Part model, mm, in its own coordinate system. Coordinates: 2 decimals unless noted, no trailing zeros. Order: outer loops, then holes, each group sorted by start corner. A loop starts at its lowest first (then second) coordinate and runs counter-clockwise, first axis right, second up.
1) Wall check: L1, parallel to Z at x = -0.5, y = 1; L2, parallel to Z at x = -1.25, y = -0.5; L3, parallel to X at y = -0.5, z = 26. Give the ranges that are in metal, low to high.
2) Cut at C-C (x = -0.5). List the corners of the cut face in (y, z), and give its area (3 significant figures).
3) Cut at D-D (y = -1.75). List the corners of the cut face in (x, z).
4) Pin check, flat tips, straight feed: pin 1 Ø0.9 at (x, y) = (2, 1) entering from +Z; pin 2 Ø1.5 at (x, y) = (1, 1) entering from -Z; pin 3 Ø1 at (y, z) = (1, 22.5) entering from +X. Stop position of each tip, or through.
5) Cut at A-A (y = 0.5). List the corners of the cut face in (x, z).
6) Cut at B-B (z = 14). List the corners of the cut face in (x, y), and give its area (3 significant figures).
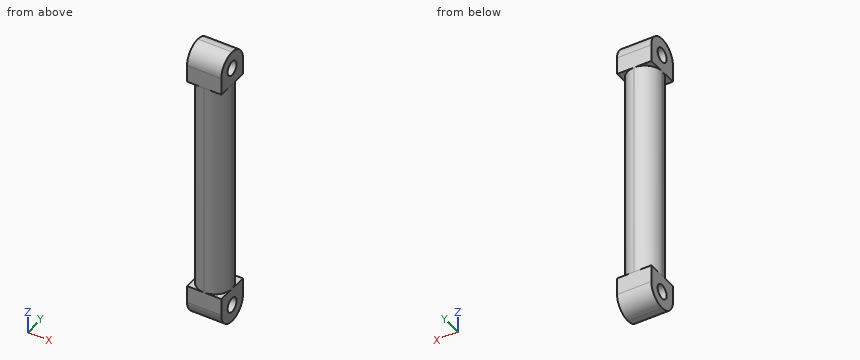
```python
from build123d import *

# Parameters (mm, degrees)
F0_R     = 1.25
F1_DEPTH = 6
F2_DEPTH = 44
F3_R     = 1.25
F4_DEPTH = 6
F5_W     = 6
F5_H     = 6
F6_DEPTH = 6
F7_R     = 1.25
F8_DEPTH = 25


# Not quite as in the source:
# - a feature names something its author has since deleted; it is built from what else it names


with BuildPart() as f1:
    # F0 (on Top) → F1 (new body)
    with BuildSketch(Plane.XY):
        with BuildLine():
            ThreePointArc((0, -3), (2.1213203436, -2.1213203436), (3, 0))
            ThreePointArc((3, 0), (2.1213203436, 2.1213203436), (0, 3))
            ThreePointArc((0, 3), (-2.1213203436, 2.1213203436), (-3, 0))
            ThreePointArc((-3, 0), (-2.1213203436, -2.1213203436), (0, -3))
        make_face()
        Circle(F0_R, mode=Mode.SUBTRACT)
        with BuildLine():
            ThreePointArc((-3, 0), (-2.1213203436, 2.1213203436), (0, 3))
            Line((0, 3), (-3, 3))
            Line((-3, 3), (-3, 0))
        make_face()
        with BuildLine():
            Line((-3, -3), (0, -3))
            ThreePointArc((0, -3), (-2.1213203436, -2.1213203436), (-3, 0))
            Line((-3, 0), (-3, -3))
        make_face()
        with BuildLine():
            Line((3, -3), (3, 0))
            ThreePointArc((3, 0), (2.1213203436, -2.1213203436), (0, -3))
            Line((0, -3), (3, -3))
        make_face()
        with BuildLine():
            ThreePointArc((0, 3), (2.1213203436, 2.1213203436), (3, 0))
            Line((3, 0), (3, 3))
            Line((3, 3), (0, 3))
        make_face()
        Circle(F0_R)
    extrude(amount=F1_DEPTH)

    # F0 (on Top) → F2 (join)
    with BuildSketch(Plane.XY):
        with BuildLine():
            ThreePointArc((0, -3), (2.1213203436, -2.1213203436), (3, 0))
            ThreePointArc((3, 0), (2.1213203436, 2.1213203436), (0, 3))
            ThreePointArc((0, 3), (-2.1213203436, 2.1213203436), (-3, 0))
            ThreePointArc((-3, 0), (-2.1213203436, -2.1213203436), (0, -3))
        make_face()
        Circle(F0_R, mode=Mode.SUBTRACT)
    extrude(amount=F2_DEPTH)

    # F3 (on face) → F4 (cut)
    with BuildSketch(Plane.YZ.offset(3)):
        with Locations((0, 3)):
            Circle(F3_R)
        with BuildLine():
            Line((-3, 0), (0, 0))
            ThreePointArc((0, 0), (-2.1213203436, 0.8786796564), (-3, 3))
            Line((-3, 3), (-3, 0))
        make_face()
        with BuildLine():
            Line((3, 0), (3, 3))
            ThreePointArc((3, 3), (2.1213203436, 0.8786796564), (0, 0))
            Line((0, 0), (3, 0))
        make_face()
    extrude(amount=-F4_DEPTH, mode=Mode.SUBTRACT)

    # F5 (on face) → F6 (join)
    with BuildSketch(Plane.XY.offset(44)):
        Rectangle(F5_W, F5_H)
    extrude(amount=F6_DEPTH)

    # F7 (on face) → F8 (cut)
    with BuildSketch(Plane.YZ.offset(3)):
        with Locations((0, 47)):
            Circle(F7_R)
        with BuildLine():
            Line((-3, 50), (-3, 47))
            ThreePointArc((-3, 47), (-2.1213203436, 49.1213203436), (0, 50))
            Line((0, 50), (-3, 50))
        make_face()
        with BuildLine():
            ThreePointArc((0, 50), (2.1213203436, 49.1213203436), (3, 47))
            Line((3, 47), (3, 50))
            Line((3, 50), (0, 50))
        make_face()
    extrude(amount=-F8_DEPTH, mode=Mode.SUBTRACT)


solid = f1.part
```
Geometry check:
1. L1: z = 0.17 to 2.25, 3.75 to 6, 44 to 46.25, 47.75 to 49.83
1. L2: z = 0.04 to 1.85, 4.15 to 45.85, 48.15 to 49.96
1. L3: x = -2.96 to -1.15, 1.15 to 2.96
2. outline: (-3, 3) arc R3 ccw to (3, 3) - (3, 6) - (2.96, 6) - (2.96, 44) - (3, 44) - (3, 47) arc R3 ccw to (-3, 47) - (-3, 44) - (-2.96, 44) - (-2.96, 6) - (-3, 6) - close; hole circle Ø2.5 at (0, 3); hole circle Ø2.5 at (0, 47); hole (-1.15, 6) - (1.15, 6) - (1.15, 44) - (-1.15, 44) - close
2. area: 192 mm2
3. outline: (-3, 0.56) - (3, 0.56) - (3, 6) - (2.44, 6) - (2.44, 44) - (3, 44) - (3, 49.44) - (-3, 49.44) - (-3, 44) - (-2.44, 44) - (-2.44, 6) - (-3, 6) - close
4. pin 1: stops at z = 49.95
4. pin 2: stops at z = 0.01
4. pin 3: stops at x = 2.96
5. outline: (-3, 0.04) - (3, 0.04) - (3, 1.85) - (-3, 1.85) - close; (-3, 4.15) - (3, 4.15) - (3, 6) - (2.96, 6) - (2.96, 44) - (3, 44) - (3, 45.85) - (-3, 45.85) - (-3, 44) - (-2.96, 44) - (-2.96, 6) - (-3, 6) - close; (-3, 48.15) - (3, 48.15) - (3, 49.96) - (-3, 49.96) - close; hole (-1.15, 6) - (1.15, 6) - (1.15, 44) - (-1.15, 44) - close
6. outline: circle Ø6 at (0, 0); hole circle Ø2.5 at (0, 0)
6. area: 23.4 mm2
